```python
from build123d import *

# Parameters (mm, degrees)
F0_R     = 3.175
F1_DEPTH = 28.448


with BuildPart() as f1:
    # F0 (on Front) → F1 (new body)
    with BuildSketch(Plane.XZ):
        with BuildLine():
            ThreePointArc((-9.4502929642, 115.490625), (-0.596483242, 104.7936951058), (9.525, 114.3))
            ThreePointArc((9.525, 114.3), (9.5063048942, 114.896483242), (9.4502929642, 115.490625))
            ThreePointArc((9.4502929642, 115.490625), (0, 123.825), (-9.4502929642, 115.490625))
        make_face()
        with Locations((0, 114.3)):
            Circle(F0_R, mode=Mode.SUBTRACT)
        with BuildLine():
            ThreePointArc((9.4502929642, 115.490625), (9.5063048942, 114.896483242), (9.525, 114.3))
            ThreePointArc((9.525, 114.3), (-0.596483242, 104.7936951058), (-9.4502929642, 115.490625))
            Line((-9.4502929642, 115.490625), (-15.7504882737, 65.484375))
            ThreePointArc((-15.7504882737, 65.484375), (0, 79.375), (15.7504882737, 65.484375))
            Line((15.7504882737, 65.484375), (9.4502929642, 115.490625))
        make_face()
        with Locations((-3.175, 100.0252)):
            Circle(F0_R, mode=Mode.SUBTRACT)
        with BuildLine():
            Line((15.0944103202, 58.583252896), (15.7504882737, 65.484375))
            ThreePointArc((15.7504882737, 65.484375), (0, 79.375), (-15.7504882737, 65.484375))
            Line((-15.7504882737, 65.484375), (-15.0944103202, 58.583252896))
            ThreePointArc((-15.0944103202, 58.583252896), (0, 47.625), (15.0944103202, 58.583252896))
        make_face()
        with Locations((0, 63.5)):
            Circle(F0_R, mode=Mode.SUBTRACT)
        with BuildLine():
            ThreePointArc((15.875, 63.5), (15.8438414904, 64.4941387366), (15.7504882737, 65.484375))
            Line((15.7504882737, 65.484375), (15.0944103202, 58.583252896))
            ThreePointArc((15.0944103202, 58.583252896), (15.6786381557, 61.0108373731), (15.875, 63.5))
        make_face()
        with BuildLine():
            Line((-15.0944103202, 58.583252896), (-15.7504882737, 65.484375))
            ThreePointArc((-15.7504882737, 65.484375), (-15.8037436669, 61.9975649401), (-15.0944103202, 58.583252896))
        make_face()
        with BuildLine():
            Line((11.1940088369, 17.5558921241), (15.0944103202, 58.583252896))
            ThreePointArc((15.0944103202, 58.583252896), (0, 47.625), (-15.0944103202, 58.583252896))
            Line((-15.0944103202, 58.583252896), (-9.525, 0))
            ThreePointArc((-9.525, 0), (-6.6138273378, 6.8544082857), (0.3401785714, 9.5189234444))
            Line((0.3401785714, 9.5189234444), (10.3957843217, 9.159565412))
            Line((10.3957843217, 9.159565412), (11.1940088369, 17.5558921241))
        make_face()
        with BuildLine():
            ThreePointArc((18.824587951, 8.8583445445), (13.1322805896, 11.560363002), (11.1940088369, 17.5558921241))
            Line((11.1940088369, 17.5558921241), (10.3957843217, 9.159565412))
            Line((10.3957843217, 9.159565412), (18.824587951, 8.8583445445))
        make_face()
        with BuildLine():
            ThreePointArc((0.3401785714, 9.5189234444), (-6.6138273378, 6.8544082857), (-9.525, 0))
            ThreePointArc((-9.525, 0), (-6.6138273378, -6.8544082857), (0.3401785714, -9.5189234444))
            ThreePointArc((0.3401785714, -9.5189234444), (6.8544082857, -6.6138273378), (9.525, 0))
            ThreePointArc((9.525, 0), (6.8544082857, 6.6138273378), (0.3401785714, 9.5189234444))
        make_face()
        Circle(F0_R, mode=Mode.SUBTRACT)
        with BuildLine():
            Line((18.824587951, 8.8583445445), (10.3957843217, 9.159565412))
            Line((10.3957843217, 9.159565412), (9.525, 0))
            Line((9.525, 0), (36.5125, 0))
            ThreePointArc((36.5125, 0), (38.9384772185, 5.7120069047), (44.7334821429, 7.9324362036))
            Line((44.7334821429, 7.9324362036), (18.824587951, 8.8583445445))
        make_face()
        with BuildLine():
            ThreePointArc((9.525, 0), (6.8544082857, -6.6138273378), (0.3401785714, -9.5189234444))
            Line((0.3401785714, -9.5189234444), (44.7334821429, -7.9324362036))
            ThreePointArc((44.7334821429, -7.9324362036), (38.9384772185, -5.7120069047), (36.5125, 0))
            Line((36.5125, 0), (9.525, 0))
        make_face()
        with BuildLine():
            ThreePointArc((52.3875, 0), (50.1620069047, 5.5115227815), (44.7334821429, 7.9324362036))
            ThreePointArc((44.7334821429, 7.9324362036), (38.9384772185, 5.7120069047), (36.5125, 0))
            ThreePointArc((36.5125, 0), (38.9384772185, -5.7120069047), (44.7334821429, -7.9324362036))
            ThreePointArc((44.7334821429, -7.9324362036), (50.1620069047, -5.5115227815), (52.3875, 0))
        make_face()
        with BuildLine():
            ThreePointArc((47.625, 0), (44.45, -3.175), (41.275, 0))
            ThreePointArc((41.275, 0), (44.45, 3.175), (47.625, 0))
        make_face(mode=Mode.SUBTRACT)
    extrude(amount=F1_DEPTH)


solid = f1.part
```
Work out the finished part from the listing and answer in its coordinate system (mm). A direction names the side the tool comes from. Give positions to 0.01 mm unless a question says otherwise; leave off trailing zeros. Loops run counter-clockwise (first coordinate to the right, second up) from the corner with the lowest first, then second, coordinate; pieces in that order, holes last. Notation, with made-up numbers: (73, 28) -> (114, 28) arc R32 cw to (114, 60) -> close; hole circle Ø8 at (79, -11). An arc over 180 degrees is marked (long way). One line per question, with ' | ' between items. Start each with the question number.
1) Each of these flat-tipped pins is pushed along its axis until it touches: pin 1 (4 mm diameter, centred on x = 24, y = -3, fed in from +Z); pin 2 (10 mm diameter, centred on x = 6.5, z = 56.5, fed in from +Y); pin 3 (6 mm diameter, centred on y = -6, z = 5, fed in from +X); pin 4 (1.5 mm diameter, centred on y = -18, z = 62, fed in from -X). Where does it stop, or does it pass through?
2) Section A-A, the plane y = -24.5 is taken. State how many separate pieces and enclosed holes the cut face has, then the cut area to 3 significant figures.
3) Section C-C, the plane z = 31 is taken. Determine the outline of the cut face in (x, y).
4) Straight lines are drawn through the part: L1, parallel to X at y = -7, z = 2.5; L2, parallel to X at y = -21.5, z = 112.5; L3, parallel to Z at x = 44.45, y = -14.5 (3 decimals). For each, find the intervals that lie inside material, in ascending order.
5) Section B-B, the plane x = 25 is taken. Determine the outline of the cut face in (y, z).
6) Determine the mould class of faces 1 (the face through (3, 0, 43)), 2 (the face through (6.925, -14.025, 6.54)), 3 (the face through (12.644, -14.025, 90.137)) for opening direction Z: +Z half, -Z half, draft (parallel to the pull), parting line (faces both ways), or undercut.
7) For faces 4 (the face through (-0.69, -14.02, 111.2)), 5 (the face through (13.192, -14.025, 11.493)), determine the directions among +Z, -Z, +X, -X, +Y, -Y from which every point of the face is accessible in a straight line to the end or side of a thin tool.
Resolved:
1) pin 1: z = 8.74 | pin 2: y = 0 | pin 3: x = 52.13 | pin 4: x = -15.86
2) separate pieces: 1 | enclosed holes: 6 | area: 3,730 mm2
3) outline: (-12.47, -28.45) -> (12.47, -28.45) -> (12.47, 0) -> (-12.47, 0) -> close
4) L1: -9.76 to -1.96, 1.96 to 9.19, 9.76 to 42.49, 46.41 to 51.98 | L2: -9.83 to -2.62, 2.62 to 9.83 | L3: -7.943 to -3.175, 3.175 to 7.943
5) outline: (-28.45, -8.64) -> (0, -8.64) -> (0, 8.64) -> (-28.45, 8.64) -> close
6) face 1: draft | face 2: undercut | face 3: +Z half
7) face 4: +Y, -Y | face 5: +X, +Y, -Y
